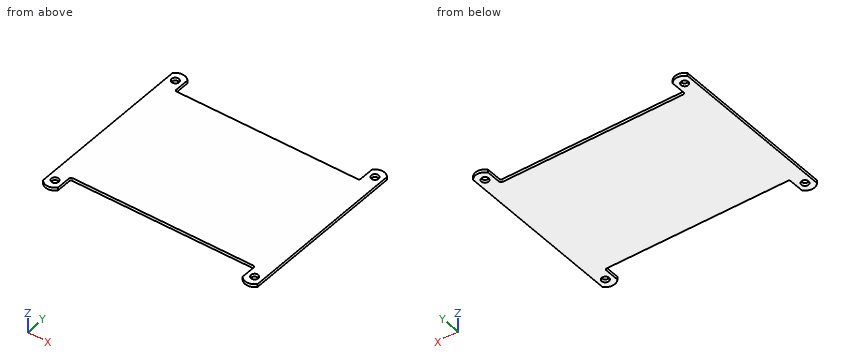
```python
from build123d import *

# Parameters (mm, degrees)
SKETCH_W                   = 104
SKETCH_H                   = 77
PAD_DEPTH                  = 1.66
SKETCH001_W                = 8.5
SKETCH001_H                = 49.76
PAD001_DEPTH               = 1.66
SKETCH002_R                = 2.05
POCKET_DEPTH               = 1.66
POCKET001_DEPTH            = 5
SKETCH001_MIRRORED_2_W     = 8.5
SKETCH001_MIRRORED_2_H     = 49.76
PAD001_MIRRORED_2_DEPTH    = 1.66
SKETCH002_MIRRORED_2_R     = 2.05
POCKET_MIRRORED_2_DEPTH    = 1.66
POCKET001_MIRRORED_2_DEPTH = 5
FILLET_R                   = 1


with BuildPart() as part:
    # Sketch → Pad (new body)
    with BuildSketch(Plane.XY):
        Rectangle(SKETCH_W, SKETCH_H)
    extrude(amount=PAD_DEPTH)

    # Sketch001 → Pad001 (join)
    with BuildSketch(Plane.XY):
        with Locations((-56.25, 24.88)):
            Rectangle(SKETCH001_W, SKETCH001_H)
    pad001 = extrude(amount=PAD001_DEPTH)

    # Sketch002 → Pocket (cut)
    with BuildSketch(Plane.XY):
        with Locations((-56.25, 44.37)):
            Circle(SKETCH002_R)
    pocket = extrude(amount=POCKET_DEPTH, mode=Mode.SUBTRACT)

    # Sketch003 → Pocket001 (cut)
    with BuildSketch(Plane.XY):
        with BuildLine():
            ThreePointArc((-52, 47.685057), (-56.25, 49.76), (-60.5, 47.685057))
            Line((-60.5, 47.685057), (-60.5, 51.185057))
            Line((-60.5, 51.185057), (-52, 51.185057))
            Line((-52, 51.185057), (-52, 47.685057))
        make_face()
    pocket001 = extrude(amount=POCKET001_DEPTH, mode=Mode.SUBTRACT)

    # Sketch001 Mirrored 2 → Pad001 Mirrored 2 (add)
    with BuildSketch(Plane(origin=(0, 0, 0), x_dir=(-1, 0, 0), z_dir=(0, 0, -1))):
        with Locations((-56.25, 24.88)):
            Rectangle(SKETCH001_MIRRORED_2_W, SKETCH001_MIRRORED_2_H)
    pad001_mirrored_2 = extrude(amount=-PAD001_MIRRORED_2_DEPTH)

    # Sketch002 Mirrored 2 → Pocket Mirrored 2 (cut)
    with BuildSketch(Plane(origin=(0, 0, 0), x_dir=(-1, 0, 0), z_dir=(0, 0, -1))):
        with Locations((-56.25, 44.37)):
            Circle(SKETCH002_MIRRORED_2_R)
    pocket_mirrored_2 = extrude(amount=-POCKET_MIRRORED_2_DEPTH, mode=Mode.SUBTRACT)

    # Sketch003 Mirrored 2 → Pocket001 Mirrored 2 (cut)
    with BuildSketch(Plane(origin=(0, 0, 0), x_dir=(-1, 0, 0), z_dir=(0, 0, -1))):
        with BuildLine():
            ThreePointArc((-52, 47.685057), (-56.25, 49.76), (-60.5, 47.685057))
            Line((-60.5, 47.685057), (-60.5, 51.185057))
            Line((-60.5, 51.185057), (-52, 51.185057))
            Line((-52, 51.185057), (-52, 47.685057))
        make_face()
    pocket001_mirrored_2 = extrude(amount=-POCKET001_MIRRORED_2_DEPTH, mode=Mode.SUBTRACT)

    # Mirrored001: Pad001, Pocket, Pocket001, Pad001 Mirrored 2, Pocket Mirrored 2, Pocket001 Mirrored 2 across XZ
    add(pad001.mirror(Plane.XZ))
    add(pocket.mirror(Plane.XZ), mode=Mode.SUBTRACT)
    add(pocket001.mirror(Plane.XZ), mode=Mode.SUBTRACT)
    add(pad001_mirrored_2.mirror(Plane.XZ))
    add(pocket_mirrored_2.mirror(Plane.XZ), mode=Mode.SUBTRACT)
    add(pocket001_mirrored_2.mirror(Plane.XZ), mode=Mode.SUBTRACT)

    # Fillet
    fillet_edges = [part.edges().sort_by_distance(p)[0] for p in [
        (-52, 38.5, 0.83),
        (52, 38.5, 0.83),
        (-52, -38.5, 0.83),
        (52, -38.5, 0.83),
    ]]
    fillet(fillet_edges, radius=FILLET_R)


solid = part.part
```
Verification items for the finished model (mm, model axes). Coordinates: 2 decimals unless noted, no trailing zeros. Write each loop counter-clockwise with the first axis right and the second up, starting at its lowest first coordinate (ties: lowest second). Pieces come first, ordered by that corner, then holes. Notation, with made-up numbers: (9.25, 37.25) - (37.25, 37.25) arc R21 ccw to (37.25, 54.25) - close; hole circle Ø10 at (75.25, 74). An arc over 180 degrees is marked (long way). Write item = value, one per line.
Q1. Cross-section at A-A (z = 0.6). Enter the section's corners in (x, y), plus the area to 3 significant figures.
Answer:
outline = (-60.5, -47.69) arc R5.39 ccw to (-52, -47.69) - (-52, -39.5) arc R1 cw to (-51, -38.5) - (51, -38.5) arc R1 cw to (52, -39.5) - (52, -47.69) arc R5.39 ccw to (60.5, -47.69) - (60.5, 47.69) arc R5.39 ccw to (52, 47.69) - (52, 39.5) arc R1 cw to (51, 38.5) - (-51, 38.5) arc R1 cw to (-52, 39.5) - (-52, 47.69) arc R5.39 ccw to (-60.5, 47.69) - close; hole circle Ø4.1 at (-56.25, -44.37); hole circle Ø4.1 at (-56.25, 44.37); hole circle Ø4.1 at (56.25, -44.37); hole circle Ø4.1 at (56.25, 44.37)
area = 9,630 mm²
Q2. Go/stop test with flat-tipped pins: pin 1 Ø4.5 at (x, y) = (56.25, 44.37) entering from +Z; pin 2 Ø0.8 at (x, z) = (8, 1) entering from -Y. Record where each tip stops, or that it passes through.
Answer:
pin_1 = 1.66
pin_2 = -38.5
Q3. Cross-section at D-D (x = 29.5). Enter the section's corners in (y, z).
Answer:
outline = (-38.5, 0) - (38.5, 0) - (38.5, 1.66) - (-38.5, 1.66) - close
Q4. Cross-section at B-B (x = 56.25). Enter the section's corners in (y, z).
Answer:
outline = (-49.76, 0) - (-46.42, 0) - (-46.42, 1.66) - (-49.76, 1.66) - close; (-42.32, 0) - (42.32, 0) - (42.32, 1.66) - (-42.32, 1.66) - close; (46.42, 0) - (49.76, 0) - (49.76, 1.66) - (46.42, 1.66) - close
Q5. Cross-section at C-C (y = -44.37). Enter the section's corners in (x, z), plus the area to 3 significant figures.
Answer:
outline = (-60.5, 0) - (-58.3, 0) - (-58.3, 1.66) - (-60.5, 1.66) - close; (-54.2, 0) - (-52, 0) - (-52, 1.66) - (-54.2, 1.66) - close; (52, 0) - (54.2, 0) - (54.2, 1.66) - (52, 1.66) - close; (58.3, 0) - (60.5, 0) - (60.5, 1.66) - (58.3, 1.66) - close
area = 14.6 mm²
Q6. Material ranges on L1, parallel to Y at x = 56.25, z = 1; L2, parallel to X at y = -44.5, z = 0.75; L3, parallel to Y at x = 41, z = 1.2, recorded low to high. Write a range as from..to.
Answer:
L1 = -49.76..-46.42, -42.32..42.32, 46.42..49.76
L2 = -60.5..-58.3, -54.2..-52, 52..54.2, 58.3..60.5
L3 = -38.5..38.5
